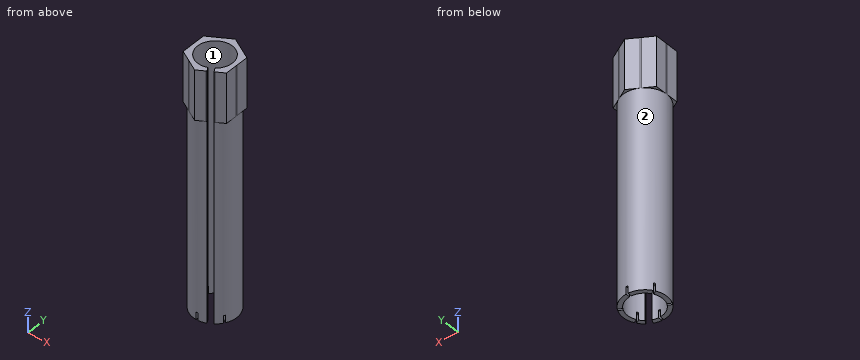
Autodesk Fusion 360 part; units mm, degrees
sketch "Sketch1" plane through (0, 0, 0) normal (0, 0, 1) x (1, 0, 0)
  circle A0 centre (0, 0) radius 10
  dimension "d1" = 20
sketch "Sketch2" plane through (0, 0, 0) normal (0, 0, 1) x (1, 0, 0)
  circle A0 centre (0, 0) radius 17.5
  circle A1 centre (0, 0) radius 14
  line L0 (-0.75, 19.1081) -> (0.75, 19.1081)
  line L1 (0.75, 19.1081) -> (0.75, -21)
  line L2 (0.75, -21) -> (-0.75, -21)
  line L3 (-0.75, -21) -> (-0.75, 19.1081)
  line L4 (0, 23) -> (0, -27)
  line L5 (-30, 0) -> (27, 0)
  line L6 (-16.3017, -8.5458) -> (18.0876, 11.3089)
  line L7 (18.0876, 11.3089) -> (18.8376, 10.0099)
  line L8 (18.8376, 10.0099) -> (-15.5517, -9.8448)
  line L9 (-15.5517, -9.8448) -> (-16.3017, -8.5458)
  line L10 (-16.8985, 10.6224) -> (17.4908, -9.2323)
  line L11 (17.4908, -9.2323) -> (16.7408, -10.5313)
  line L12 (16.7408, -10.5313) -> (-17.6485, 9.3234)
  line L13 (-17.6485, 9.3234) -> (-16.8985, 10.6224)
  line L14 (8.0661, -18.0086) -> (4.1738, -11.2669)
  line L15 (4.1738, -11.2669) -> (8.0709, -9.0169)
  line L16 (8.0709, -9.0169) -> (11.9633, -15.7586)
  line L17 (11.9633, -15.7586) -> (8.0661, -18.0086)
  dimension "d2" = 35
  dimension "d3" = 28
  dimension "d4" = 1.5
  dimension "d5" = 0.75
  dimension "d7" = 1.5
  dimension "d8" = 120
  dimension "d9" = 0.75
  dimension "d10" = 1.5
  dimension "d11" = 60
  dimension "d16" = 4.5
  dimension "d17" = 30
  dimension "d19" = 0.75
extrude "Extrude1" add sketch "Sketch2" along normal blind 200 contours A0 A1 L5 L8 | A0 A1 L5 L10 | A0 A1 L6 L8 | A0 A1 L10 L12 | A0 A1 L1 L6 | A0 A1 L12 L16 | A0 A1 L1 L4 | A0 A1 L3 L4 | A0 A1 L1 L14 | A0 A1 L3 L10 | A0 A1 L1 L4 | A0 A1 L3 L4 | A0 A1 L10 L12 | A0 A1 L3 L8 | A0 A1 L6 L8 | A0 A1 L5 L12 | A0 A1 L5 L6
extrude "Extrude2" cut sketch "Sketch2" along normal blind 6 contours A0 A1 L6 L8 | A0 A1 L10 L12 | A0 A1 L1 L4 | A0 A1 L3 L4 | A0 A1 L1 L4 | A0 A1 L3 L4 | A0 A1 L10 L12 | A0 A1 L6 L8
sketch "Sketch3" plane through (0, 0, 200) normal (0, 0, 1) x (-1, 0, 0)
  arc A0 (-10.8104, 13.7617) -> (-6.9432, 16.0637) centre (0, 0) ccw
  line L0 (-6.9432, 16.0637) -> (-5.1785, 13.007)
  arc A1 (-9.038, 10.6918) -> (-5.1785, 13.007) centre (0, 0) ccw
  line L1 (-9.038, 10.6918) -> (-10.8104, 13.7617)
  line L2 (-17.6603, 9.8038) -> (-17.3205, -10.3923)
  line L3 (-17.3205, -10.3923) -> (0.3397, -20.1962)
  line L4 (0.3397, -20.1962) -> (17.6603, -9.8038)
  line L5 (17.6603, -9.8038) -> (17.3205, 10.3923)
  line L6 (17.3205, 10.3923) -> (-0.3397, 20.1962)
  line L7 (-0.3397, 20.1962) -> (-17.6603, 9.8038)
  line L8 (-6.6088, 16.4347) -> (-6.9432, 16.0637)
  line L9 (-10.8104, 13.7617) -> (-11.4119, 13.5528)
extrude "Extrude3" add sketch "Sketch3" against normal blind 40 contours A0 L2 L7 L9 | A0 L2 L3 | A0 L6 L7 L8 | A0 L3 L4 | A0 L5 L6 | A0 L4 L5
CAD build for the part. Positions are in the model's coordinates, mm. Face numbers are marked on the shaded views. Give positions to 0.01 mm unless a question says otherwise; leave off trailing zeros. Write each loop counter-clockwise with the first axis right and the second up, starting at its lowest first coordinate (ties: lowest second). Pieces come first, ordered by that corner, then holes. Notation, with made-up numbers: (35, 16.5) -> (70, 16.5) arc R23 ccw to (70, 25.5) -> close; hole circle Ø8 at (16.5, 15). An arc over 180 degrees is marked (long way). Write each question's results on one line, items separated by ' | '.
1. Cut at D-D, the plane z = 28.5. Write the cut outline in (x, y), then the cut area to 3 significant figures.
Geometry check:
outline: (5.18, -13.01) arc R14 cw (long way) to (9.04, -10.69) -> (10.81, -13.76) arc R17.5 ccw (long way) to (6.94, -16.06) -> close | area: 331 mm²
2. Cut at A-A, the plane y = -4. Write the cut outline in (x, z), then the cut area to 3 significant figures.
Geometry check:
outline: (-17.43, 160) -> (-17.04, 160) -> (-17.04, 0) -> (-13.42, 0) -> (-13.42, 200) -> (-17.43, 200) -> close; (13.42, 0) -> (17.04, 0) -> (17.04, 160) -> (17.56, 160) -> (17.56, 200) -> (13.42, 200) -> close | area: 1,480 mm²
3. Cut at B-B, the plane x = -4. Write the cut outline in (y, z).
Geometry check:
outline: (-17.79, 160) -> (-17.04, 160) -> (-17.04, 0) -> (-13.42, 0) -> (-13.42, 200) -> (-17.79, 200) -> close; (13.42, 0) -> (17.04, 0) -> (17.04, 160) -> (18, 160) -> (18, 200) -> (13.42, 200) -> close
4. Drop flat-ended pins along their axis: P1, Ø1, axis at x = 8.5, z = 63, coming from the +Y side; P2, Ø3, axis at y = 0, z = 66.5, coming from the -X side; P3, Ø17, axis at x = 0, y = 0, coming from the +Z side; P4, Ø4, axis at y = -12.5, z = 165, coming from the -X side. Give the stop position or say it passes through.
Geometry check:
P1: y = 15.56 | P2: x = -17.5 | P3: through | P4: x = -17.13
5. Cut at C-C, the plane z = 187. Write the cut outline in (x, y), then the cut area to 3 significant figures.
Geometry check:
outline: (-17.66, 9.8) -> (-17.5, 0.21) arc R17.5 ccw to (-17.48, -0.8) -> (-17.32, -10.39) -> (-8.93, -15.05) arc R17.5 ccw to (-8.05, -15.54) -> (0.34, -20.2) -> (6.61, -16.43) -> (6.94, -16.06) -> (5.18, -13.01) arc R14 cw (long way) to (9.04, -10.69) -> (10.81, -13.76) -> (11.41, -13.55) -> (17.66, -9.8) -> (17.5, -0.2) arc R17.5 ccw to (17.48, 0.79) -> (17.32, 10.39) -> (8.92, 15.05) arc R17.5 ccw to (8.06, 15.53) -> (-0.34, 20.2) -> (-8.57, 15.26) arc R17.5 ccw to (-9.43, 14.74) -> close | area: 428 mm²
6. Two-plate mould, pull along Y, no slides. Class the marked faces 1 and 2: pulls with the +Y half, pulls with the -Y half, needs draft (parallel to the pull), parting line crosses it, or undercut.
Geometry check:
face 1: undercut | face 2: parting line crosses it
7. Wall check: probe 1 along X at (y, z) = (0, 145); probe 2 along Z at (x, y) = (3, -17.5). Give the ranges that are in metal, low to high. Write a range as [from, to].
Geometry check:
probe 1: [-17.5, -14], [14, 17.5] | probe 2: [160, 200]
